Can you work these out from the model? Positions are in its coordinate system, mm. Round coordinates to 2 decimals unless told otherwise and drop trailing zeros. Order: outer loops, then holes, each group sorted by start corner. A loop starts at its lowest first (then second) coordinate and runs counter-clockwise, first axis right, second up. Notation, with made-up numbers: (20.25, -33) -> (79.25, -33) arc R19 ccw to (79.25, -26) -> close; hole circle Ø7 at (-18.75, 31). An arc over 180 degrees is marked (long way). Use a Markdown table: item, result. Add a question column.
Q1. If we section it at C-C on x = -15.5: List the corners of the cut face in (y, z) for me.
Q2. If we section it at D-D on z = 1.45: Give the number of separate pieces and of enclosed holes in the cut face, plus the area to 3 significant figures.
Q3. We'd pull the mould along Y, two halves only. Please class faces 1 (the face through (-34.574, -11.552, 1.479)), 2 (the face through (-11, 19.75, 1)), 3 (the face through (11.923, 3.755, 1.479)), 4 (the face through (-12, 5, 3)): +Y half, -Y half, draft (parallel to the pull), parting line (faces both ways), or undercut.
Q4. I need wall thicknesses on line 1 along Y through (x, z) = (-32.55, 1.1); line 2 along Y through (x, z) = (-15.5, 1.15); line 3 along X through (y, z) = (-1, 2.3). Which ranges of each line are inside material? Lowest first, please. Write a range as [from, to].
Q5. If we section it at B-B on y = 10: List the corners of the cut face in (x, z) for me.
Q6. If we section it at A-A on x = -32.55: List the corners of the cut face in (y, z) for me, plus the area to 3 significant figures.
```python
from build123d import *

# Parameters (mm, degrees)
F0_R     = 2.55
F0_R_2   = 1.55
F0_R_3   = 12.5
F1_DEPTH = 3


with BuildPart() as f1:
    # F0 (on Top) → F1 (new body)
    with BuildSketch(Plane.XY):
        with BuildLine():
            ThreePointArc((19.75, 15.75), (18.578427, 18.578427), (15.75, 19.75))
            Line((15.75, 19.75), (-38.55, 19.75))
            ThreePointArc((-38.55, 19.75), (-41.378427, 18.578427), (-42.55, 15.75))
            Line((-42.55, 15.75), (-42.55, -15.75))
            ThreePointArc((-42.55, -15.75), (-41.378427, -18.578427), (-38.55, -19.75))
            Line((-38.55, -19.75), (15.75, -19.75))
            ThreePointArc((15.75, -19.75), (18.578427, -18.578427), (19.75, -15.75))
            Line((19.75, -15.75), (19.75, 15.75))
        make_face()
        with Locations((-32.55, -10)):
            Circle(F0_R, mode=Mode.SUBTRACT)
        with Locations((-15.5, -15.5)):
            Circle(F0_R_2, mode=Mode.SUBTRACT)
        with Locations((15.5, -15.5)):
            Circle(F0_R_2, mode=Mode.SUBTRACT)
        with Locations((-32.55, 0)):
            Circle(F0_R, mode=Mode.SUBTRACT)
        with Locations((-32.55, 10)):
            Circle(F0_R, mode=Mode.SUBTRACT)
        with Locations((-15.5, 15.5)):
            Circle(F0_R_2, mode=Mode.SUBTRACT)
        Circle(F0_R_3, mode=Mode.SUBTRACT)
        with Locations((15.5, 15.5)):
            Circle(F0_R_2, mode=Mode.SUBTRACT)
    extrude(amount=F1_DEPTH)


solid = f1.part
```
Answer below:
| question | item | result |
|---|---|---|
| 1 | outline | (-19.75, 0) -> (-17.05, 0) -> (-17.05, 3) -> (-19.75, 3) -> close; (-13.95, 0) -> (13.95, 0) -> (13.95, 3) -> (-13.95, 3) -> close; (17.05, 0) -> (19.75, 0) -> (19.75, 3) -> (17.05, 3) -> close |
| 2 | separate pieces | 1 |
| 2 | enclosed holes | 8 |
| 2 | area | 1,860 mm² |
| 3 | face 1 | undercut |
| 3 | face 2 | +Y half |
| 3 | face 3 | undercut |
| 3 | face 4 | draft |
| 4 | line 1 | [-19.75, -12.55], [-7.45, -2.55], [2.55, 7.45], [12.55, 19.75] |
| 4 | line 2 | [-19.75, -17.05], [-13.95, 13.95], [17.05, 19.75] |
| 4 | line 3 | [-42.55, -34.9], [-30.2, -12.46], [12.46, 19.75] |
| 5 | outline | (-42.55, 0) -> (-35.1, 0) -> (-35.1, 3) -> (-42.55, 3) -> close; (-30, 0) -> (-7.5, 0) -> (-7.5, 3) -> (-30, 3) -> close; (7.5, 0) -> (19.75, 0) -> (19.75, 3) -> (7.5, 3) -> close |
| 6 | outline | (-19.75, 0) -> (-12.55, 0) -> (-12.55, 3) -> (-19.75, 3) -> close; (-7.45, 0) -> (-2.55, 0) -> (-2.55, 3) -> (-7.45, 3) -> close; (2.55, 0) -> (7.45, 0) -> (7.45, 3) -> (2.55, 3) -> close; (12.55, 0) -> (19.75, 0) -> (19.75, 3) -> (12.55, 3) -> close |
| 6 | area | 72.6 mm² |
